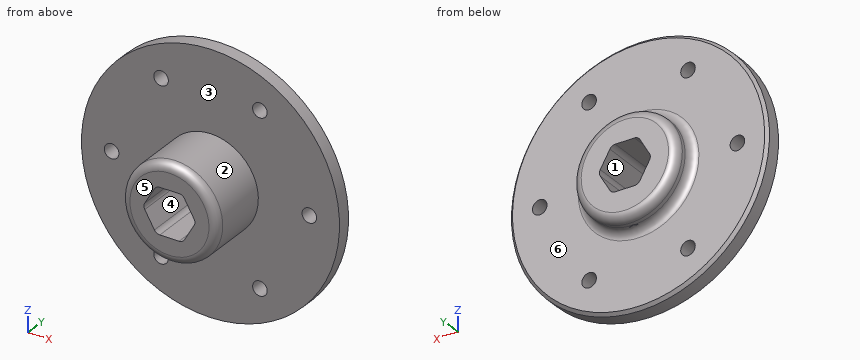
```python
from build123d import *

# Parameters (mm, degrees)
SKETCH1_R           = 31
SKETCH1_R_2         = 1.75
BOSS_EXTRUDE1_DEPTH = 4
SKETCH2_R           = 12.5
BOSS_EXTRUDE2_DEPTH = 5
CUT_EXTRUDE1_DEPTH  = 45.754888001
FILLET1_R           = 2
FILLET2_R           = 2
SKETCH5_R           = 1.6
CUT_EXTRUDE2_DEPTH  = 10
CHAMFER2_SIZE       = 0.7
SKETCH6_R           = 11.5
BOSS_EXTRUDE3_DEPTH = 15
FILLET3_R           = 2
CUT_EXTRUDE3_DEPTH  = 50.979995998
FILLET4_R           = 1.5


with BuildPart() as part:
    # Sketch1 → Boss-Extrude1 (new body)
    with BuildSketch(Plane(origin=(0, 0, 0), x_dir=(1, 0, 0), z_dir=(0, 1, 0))):
        with Locations(Location((0, 0, 0), (0, 0, 270))):
            Circle(SKETCH1_R)
        with Locations(Location((-11.875, 20.56810334, 0), (0, 0, 270))):
            Circle(SKETCH1_R_2, mode=Mode.SUBTRACT)
        with Locations(Location((11.875, 20.56810334, 0), (0, 0, 270))):
            Circle(SKETCH1_R_2, mode=Mode.SUBTRACT)
        with Locations(Location((23.75, 0, 0), (0, 0, 270))):
            Circle(SKETCH1_R_2, mode=Mode.SUBTRACT)
        with Locations(Location((11.875, -20.56810334, 0), (0, 0, 270))):
            Circle(SKETCH1_R_2, mode=Mode.SUBTRACT)
        with Locations(Location((-11.875, -20.56810334, 0), (0, 0, 270))):
            Circle(SKETCH1_R_2, mode=Mode.SUBTRACT)
        with Locations(Location((-23.75, 0, 0), (0, 0, 270))):
            Circle(SKETCH1_R_2, mode=Mode.SUBTRACT)
    extrude(amount=BOSS_EXTRUDE1_DEPTH)

    # Sketch2 → Boss-Extrude2 (add)
    with BuildSketch(Plane(origin=(0, 4, 0), x_dir=(1, 0, 0), z_dir=(0, 1, 0))):
        with Locations(Location((0, 0, 0), (0, 0, 270))):
            Circle(SKETCH2_R)
    extrude(amount=BOSS_EXTRUDE2_DEPTH)

    # Sketch3 → Cut-Extrude1 (cut, through all)
    with BuildSketch(Plane(origin=(0, 9, 0), x_dir=(1, 0, 0), z_dir=(0, 1, 0))):
        Polygon((3.175426481, 5.5), (-3.175426481, 5.5), (-6.350852961, 0), (-3.175426481, -5.5), (3.175426481, -5.5), (6.350852961, 0), align=None)
    extrude(amount=-CUT_EXTRUDE1_DEPTH, mode=Mode.SUBTRACT)

    # Fillet1
    fillet1_edges = [part.edges().sort_by_distance(p)[0] for p in [
        (3.175426481, 4.5, -5.5),
        (6.350852961, 4.5, 0),
        (3.175426481, 4.5, 5.5),
        (-3.175426481, 4.5, 5.5),
        (-6.350852961, 4.5, 0),
        (-3.175426481, 4.5, -5.5),
    ]]
    fillet(fillet1_edges, radius=FILLET1_R)

    # Fillet2
    fillet2_edges = [part.edges().sort_by_distance(p)[0] for p in [
        (0, 4, -12.5),
        (0, 9, -12.5),
    ]]
    fillet(fillet2_edges, radius=FILLET2_R)

    # Sketch5 → Cut-Extrude2 (cut)
    with BuildSketch(Plane(origin=(0, 9, -12.5), x_dir=(-1, 0, 0), z_dir=(0, 0, -1))):
        with Locations((0, -4.5)):
            Circle(SKETCH5_R)
    extrude(amount=-CUT_EXTRUDE2_DEPTH, mode=Mode.SUBTRACT)

    # Chamfer2
    chamfer2_edges = [part.edges().sort_by_distance(p)[0] for p in [
        (0, 4, -31),
    ]]
    chamfer(chamfer2_edges, length=CHAMFER2_SIZE)

    # Sketch6 → Boss-Extrude3 (add)
    with BuildSketch(Plane(origin=(0, 0, 0), x_dir=(-1, 0, 0), z_dir=(0, -1, 0))):
        with Locations(Location((0, 0, 0), (0, 0, 270))):
            Circle(SKETCH6_R)
    extrude(amount=BOSS_EXTRUDE3_DEPTH)

    # Fillet3
    fillet3_edges = [part.edges().sort_by_distance(p)[0] for p in [
        (0, -15, -11.5),
    ]]
    fillet(fillet3_edges, radius=FILLET3_R)

    # Sketch7 → Cut-Extrude3 (cut, through all)
    with BuildSketch(Plane(origin=(0, -15, 0), x_dir=(-1, 0, 0), z_dir=(0, -1, 0))):
        Polygon((-3.175426481, -5.5), (3.175426481, -5.5), (6.350852961, 0), (3.175426481, 5.5), (-3.175426481, 5.5), (-6.350852961, 0), align=None)
    extrude(amount=-CUT_EXTRUDE3_DEPTH, mode=Mode.SUBTRACT)

    # Fillet4
    fillet4_edges = [part.edges().sort_by_distance(p)[0] for p in [
        (3.175426481, -3, 5.5),
        (3.175426481, -3, -5.5),
        (6.350852961, -3, 0),
        (-3.175426481, -3, -5.5),
        (-6.350852961, -3, 0),
        (-3.175426481, -3, 5.5),
    ]]
    fillet(fillet4_edges, radius=FILLET4_R)


solid = part.part
```
Source: CAD feature listing. Evaluate the final solid. Frame: model axes, mm. Face numbers are marked on the shaded views. A direction names the side the tool comes from. Coordinates: 2 decimals unless noted, no trailing zeros. Loops run counter-clockwise (first coordinate to the right, second up) from the corner with the lowest first, then second, coordinate; pieces in that order, holes last. Notation, with made-up numbers: (42.25, 36) - (59.25, 36) arc R19 ccw to (59.25, 57) - close; hole circle Ø8 at (51, -39). An arc over 180 degrees is marked (long way). Answer as CSV lines item,"result".
1. Section B-B (z = 21.5). Count the separate pieces of the cut face and the enclosed holes in it, then the cut area to 3 significant figures.
Established:
separate pieces,"3"
enclosed holes,"0"
area,"154 mm2"
2. Contact query for flat-ended pins moving along their axis: pin 1 (2 mm diameter, centred on x = -11.88, z = 20.57, fed in from +Y); pin 2 (4 mm diameter, centred on y = -8.5, z = 0.5, fed in from -X); pin 3 (5.5 mm diameter, centred on x = 11.88, z = 20.57, fed in from -Y); pin 4 (8 mm diameter, centred on x = 14.5, y = 5.5, fed in from +Z). Output: stop coordinate, or through.
Established:
pin 1,"passes through"
pin 2,"stops at x = -11.5"
pin 3,"stops at y = 0"
pin 4,"stops at z = 28.92"
3. Ray query, line 1 (Z direction, x = -1, y = 0.75); line 2 (Z direction, x = -11, y = 2.25); line 3 (X direction, y = 2, z = 6.5). Return the intervals inside material, ascending.
Established:
line 1,"z = -30.98 to -5.5, 5.5 to 30.98"
line 2,"z = -28.98 to -22.08, -19.05 to 19.05, 22.08 to 28.98"
line 3,"x = -30.31 to 30.31"
4. Mould query, pull axis Z, two halves, no side actions, for the marked faces 1, 2 and 3. Classes: released by +Z, released by -Z, zero draft, split by the parting line, or undercut.
Established:
face 1,"undercut"
face 2,"split by the parting line"
face 3,"zero draft"
5. Reachability of the marked faces 4, 5 and 6 from +Z, -Z, +X, -X, +Y, -Y: full face, straight path, thin tool, end or side. Return the list, or none.
Established:
face 4,"+Y, -Y"
face 5,"+Z, -Z, +X, -X, -Y"
face 6,"+Y"
6. Section A-A (y = -9.75). Return loops of the section in (x, z), then the cut area to 3 significant figures.
Established:
outline,"circle Ø23 at (0, 0); hole (-5.92, -0.75) - (-3.61, -4.75) arc R1.5 ccw to (-2.31, -5.5) - (2.31, -5.5) arc R1.5 ccw to (3.61, -4.75) - (5.92, -0.75) arc R1.5 ccw to (5.92, 0.75) - (3.61, 4.75) arc R1.5 ccw to (2.31, 5.5) - (-2.31, 5.5) arc R1.5 ccw to (-3.61, 4.75) - (-5.92, 0.75) arc R1.5 ccw to start"
area,"311 mm2"
